Input: part model. Units: mm. Frame: model coordinates. Face numbers are marked on the shaded views. A direction names the side the tool comes from. Coordinates: 2 decimals unless noted, no trailing zeros. Loops run counter-clockwise (first coordinate to the right, second up) from the corner with the lowest first, then second, coordinate; pieces in that order, holes last. Notation, with made-up numbers: (-18, 14) - (7, 14) arc R32 ccw to (7, 40) - close; hole circle Ø4 at (68, -15). An arc over 180 degrees is marked (long way). Use one line per item in the form item = value.
Autodesk Inventor part; units mm, degrees
ref_plane "YZ Plane" through (0, 0, 0) normal (1, 0, 0) x (0, 1, 0)
ref_plane "XZ Plane" through (0, 0, 0) normal (0, 1, 0) x (-1, 0, 0)
ref_plane "XY Plane" through (0, 0, 0) normal (0, 0, 1) x (1, 0, 0)
sketch "Sketch1" plane through (0, 0, 0) normal (0, 0, 1) x (1, 0, 0)
  circle A0 centre (0, 0) radius 5
  dimension "d0" = 10
extrude "Extrusion1" add sketch "Sketch1" along normal blind 2
sketch "Sketch2" plane through (0, 0, 2) normal (0, 0, 1) x (1, 0, 0)
  circle A0 centre (0, 0) radius 3.75
  circle A1 centre (0, 0) radius 2.1875
  dimension "d3" = 7.5
  dimension "d4" = 4.375
extrude "Extrusion2" add sketch "Sketch2" along normal blind 3.5
sketch "Sketch3" plane through (0, 0, 0) normal (0, 0, -1) x (-1, 0, 0)
  circle A0 centre (0, 0) radius 2.1875
extrude "Extrusion3" cut sketch "Sketch3" against normal blind 2.5
fillet "Face Fillet1" radius 0.5 1 edges at (-3.75, 0, 2)
properties part number "hombrocojinete"
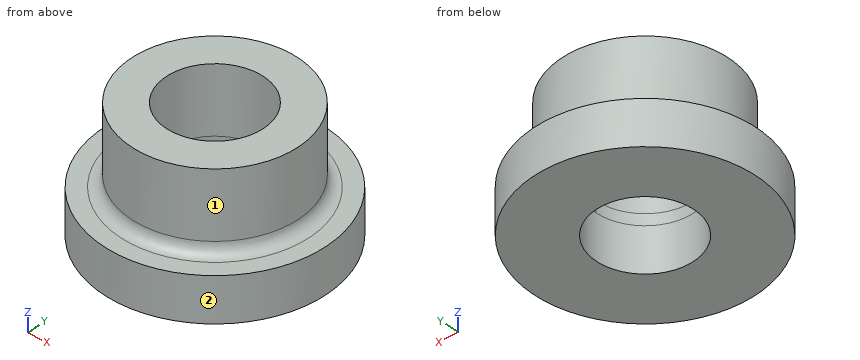
Q1. Cut plane B-B, the plane z = 0.8. Return loops of the section in (x, y) (1 decimal), then the cut area to 3 significant figures.
Check values:
outline = circle Ø10 at (0, 0); hole circle Ø4.4 at (0, 0)
area = 63.5 mm²
Q2. Ray query, line 1 along Y through (x, z) = (0, 0.5); line 2 along Y through (x, z) = (0, 4.75); line 3 along X through (y, z) = (2, 4.7). Return the intervals inside material, ascending. Write a range as [from, to].
Check values:
line_1 = [-5, -2.19], [2.19, 5]
line_2 = [-3.75, -2.19], [2.19, 3.75]
line_3 = [-3.17, -0.89], [0.89, 3.17]
Q3. Set-up query: the marked faces 1 and 2. Return all of +Z, -Z, +X, -X, +Y, -Y with unobstructed straight access to the full face (end or side cutting, diameter ignored); none if empty.
Check values:
face_1 = +Z
face_2 = +Z, -Z
Q4. First-contact query: P1, Ø1.5, axis at y = -2, z = 3, coming from the -X side; P2, Ø2, axis at y = -2.5, z = 2.5, coming from the +X side. Flat tips, straight axial feed; report the tip coordinate or a pass-through.
Check values:
P1 = -3.54
P2 = 4.73
Q5. Cut plane A-A, the plane x = 0. Return loops of the section in (y, z), then the cut area to 3 significant figures.
Check values:
outline = (-5, 0) - (-2.19, 0) - (-2.19, 5.5) - (-3.75, 5.5) - (-3.75, 2.5) arc R0.5 cw to (-4.25, 2) - (-5, 2) - close; (2.19, 0) - (5, 0) - (5, 2) - (4.25, 2) arc R0.5 cw to (3.75, 2.5) - (3.75, 5.5) - (2.19, 5.5) - close
area = 22.3 mm²
